```python
from build123d import *

# Parameters (mm, degrees)
F0_W     = 12
F0_H     = 12
F1_DEPTH = 82
F3_D     = 5
F3_DEPTH = 20
F3_TIP   = 1.5021515476
F5_D     = 5
F5_DEPTH = 20
F5_TIP   = 1.5021515476


with BuildPart() as f1:
    # F0 (on Top) → F1 (new body)
    with BuildSketch(Plane.XY):
        Rectangle(F0_W, F0_H)
    extrude(amount=-F1_DEPTH)

    # F3
    with Locations(Plane.XY):
        with Locations((0, 0)):
            Hole(F3_D / 2, depth=F3_DEPTH)
            with Locations((0, 0, -(F3_DEPTH + F3_TIP / 2))):  # 118° drill point
                Cone(0, F3_D / 2, F3_TIP, mode=Mode.SUBTRACT)

    # F5
    with Locations(Plane(origin=(0, 0, -82), x_dir=(1, 0, 0), z_dir=(0, 0, -1))):
        with Locations((0, 0)):
            Hole(F5_D / 2, depth=F5_DEPTH)
            with Locations((0, 0, -(F5_DEPTH + F5_TIP / 2))):  # 118° drill point
                Cone(0, F5_D / 2, F5_TIP, mode=Mode.SUBTRACT)


solid = f1.part
```
Model file for the job. Use its own axes, mm. A direction names the side the tool comes from. Coordinates: 2 decimals unless noted, no trailing zeros. Loops run counter-clockwise (first coordinate to the right, second up) from the corner with the lowest first, then second, coordinate; pieces in that order, holes last. Notation, with made-up numbers: (63.25, -2) -> (113.25, -2) arc R29 cw to (113.25, 25) -> close; hole circle Ø8 at (79.25, 0). An arc over 180 degrees is marked (long way). Answer as a JSON object with one key per item and string values.
Q1. Cut at A-A (z = -74). List the corners of the cut face in (x, y), and give its area (3 significant figures).
Report:
{"outline": "(-6, -6) -> (6, -6) -> (6, 6) -> (-6, 6) -> close; hole circle Ø5 at (0, 0)", "area": "124 mm2"}
Q2. 3-axis set-ups, long thin cutter, end or side, ignore diameter. For faces 1 (the cylindrical face through (0.54, 2.44, -71.86)), 2 (the cylindrical face through (0.54, -2.44, -10.14)), 3 (the flat face through (-6, 0, -40)): which of +Z, -Z, +X, -X, +Y, -Y reach the whole face in a straight line?
Report:
{"face 1": "-Z", "face 2": "+Z", "face 3": "+Z, -Z, -X, +Y, -Y"}
Q3. Pull direction Y, two halves, no side cores. Call faces 4 (the conical face through (-0.094, -0.424, -21.241)), 5 (the flat face through (3, 0, 0)), 6 (the flat face through (0, -6, -40)): released by +Y, released by -Y, zero draft, split by the parting line, or undercut.
Report:
{"face 4": "undercut", "face 5": "zero draft", "face 6": "released by -Y"}
Q4. Probe probe 1 along Y at (x, z) = (0, -11); probe 2 along Z at (x, y) = (0.75, 0.5). List the from-to ranges inside material, lowest first.
Report:
{"probe 1": "y = -6 to -2.5, 2.5 to 6", "probe 2": "z = -61.04 to -20.96"}
Q5. Flat gauge pin, fed straight in: P1, Ø4, axis at x = 0, y = 0, coming from the +Z side. Where does the tip first touch, or does it go through?
Report:
{"P1": "stops at z = -20.3"}
